from build123d import *

# Parameters (mm, degrees)
SKETCH1_R                 = 2.1
BOSS_EXTRUDE1_DEPTH       = 500
M5X0_8_TAPPED_HOLE1_D     = 4.2
M5X0_8_TAPPED_HOLE1_DEPTH = 13.97
M5X0_8_TAPPED_HOLE1_TIP   = 1.2618073
M5X0_8_TAPPED_HOLE2_D     = 4.2
M5X0_8_TAPPED_HOLE2_DEPTH = 13.97
M5X0_8_TAPPED_HOLE2_TIP   = 1.2618073


with BuildPart() as part:
    # Sketch1 → Boss-Extrude1 (new body)
    with BuildSketch(Plane(origin=(0, 0, 0), x_dir=(-1, 0, 0), z_dir=(0, 0, -1))):
        with BuildLine():
            Line((-3.9, -0.21), (-3.9, -2.839339828))
            Line((-3.9, -2.839339828), (-6.560660172, -5.5))
            Line((-6.560660172, -5.5), (-8.2, -5.5))
            Line((-8.2, -5.5), (-8.2, -3.125))
            Line((-8.2, -3.125), (-8.545, -3.125))
            Line((-8.545, -3.125), (-10, -4.58))
            Line((-10, -4.58), (-10, -9.5))
            ThreePointArc((-10, -9.5), (-9.853553391, -9.853553391), (-9.5, -10))
            Line((-9.5, -10), (-4.58, -10))
            Line((-4.58, -10), (-3.125, -8.545))
            Line((-3.125, -8.545), (-3.125, -8.2))
            Line((-3.125, -8.2), (-5.5, -8.2))
            Line((-5.5, -8.2), (-5.5, -6.560660172))
            Line((-5.5, -6.560660172), (-2.839339828, -3.9))
            Line((-2.839339828, -3.9), (-0.21, -3.9))
            Line((-0.21, -3.9), (0, -3.69))
            Line((0, -3.69), (0.21, -3.9))
            Line((0.21, -3.9), (2.839339828, -3.9))
            Line((2.839339828, -3.9), (5.5, -6.560660172))
            Line((5.5, -6.560660172), (5.5, -8.2))
            Line((5.5, -8.2), (3.125, -8.2))
            Line((3.125, -8.2), (3.125, -8.545))
            Line((3.125, -8.545), (4.58, -10))
            Line((4.58, -10), (9.5, -10))
            ThreePointArc((9.5, -10), (9.853553391, -9.853553391), (10, -9.5))
            Line((10, -9.5), (10, -4.58))
            Line((10, -4.58), (8.545, -3.125))
            Line((8.545, -3.125), (8.2, -3.125))
            Line((8.2, -3.125), (8.2, -5.5))
            Line((8.2, -5.5), (6.560660172, -5.5))
            Line((6.560660172, -5.5), (3.9, -2.839339828))
            Line((3.9, -2.839339828), (3.9, -0.21))
            Line((3.9, -0.21), (3.69, 0))
            Line((3.69, 0), (3.9, 0.21))
            Line((3.9, 0.21), (3.9, 2.839339828))
            Line((3.9, 2.839339828), (6.560660172, 5.5))
            Line((6.560660172, 5.5), (8.2, 5.5))
            Line((8.2, 5.5), (8.2, 3.125))
            Line((8.2, 3.125), (8.545, 3.125))
            Line((8.545, 3.125), (10, 4.58))
            Line((10, 4.58), (10, 9.5))
            ThreePointArc((10, 9.5), (9.853553391, 9.853553391), (9.5, 10))
            Line((9.5, 10), (4.58, 10))
            Line((4.58, 10), (3.125, 8.545))
            Line((3.125, 8.545), (3.125, 8.2))
            Line((3.125, 8.2), (5.5, 8.2))
            Line((5.5, 8.2), (5.5, 6.560660172))
            Line((5.5, 6.560660172), (2.839339828, 3.9))
            Line((2.839339828, 3.9), (0.21, 3.9))
            Line((0.21, 3.9), (0, 3.69))
            Line((0, 3.69), (-0.21, 3.9))
            Line((-0.21, 3.9), (-2.839339828, 3.9))
            Line((-2.839339828, 3.9), (-5.5, 6.560660172))
            Line((-5.5, 6.560660172), (-5.5, 8.2))
            Line((-5.5, 8.2), (-3.125, 8.2))
            Line((-3.125, 8.2), (-3.125, 8.545))
            Line((-3.125, 8.545), (-4.58, 10))
            Line((-4.58, 10), (-9.5, 10))
            ThreePointArc((-9.5, 10), (-9.853553391, 9.853553391), (-10, 9.5))
            Line((-10, 9.5), (-10, 4.58))
            Line((-10, 4.58), (-8.545, 3.125))
            Line((-8.545, 3.125), (-8.2, 3.125))
            Line((-8.2, 3.125), (-8.2, 5.5))
            Line((-8.2, 5.5), (-6.560660172, 5.5))
            Line((-6.560660172, 5.5), (-3.9, 2.839339828))
            Line((-3.9, 2.839339828), (-3.9, 0.21))
            Line((-3.9, 0.21), (-3.69, 0))
            Line((-3.69, 0), (-3.9, -0.21))
        make_face()
        Circle(SKETCH1_R, mode=Mode.SUBTRACT)
    extrude(amount=-BOSS_EXTRUDE1_DEPTH)

    # Split1
    split(bisect_by=Plane.XY.offset(68.2), keep=Keep.TOP)

    # M5x0.8 Tapped Hole1
    with Locations(Plane.XY.offset(500)):
        with Locations((0, 0)):
            Hole(M5X0_8_TAPPED_HOLE1_D / 2, depth=M5X0_8_TAPPED_HOLE1_DEPTH)
            with Locations((0, 0, -(M5X0_8_TAPPED_HOLE1_DEPTH + M5X0_8_TAPPED_HOLE1_TIP / 2))):  # 118° drill point
                Cone(0, M5X0_8_TAPPED_HOLE1_D / 2, M5X0_8_TAPPED_HOLE1_TIP, mode=Mode.SUBTRACT)

    # M5x0.8 Tapped Hole2
    with Locations(Plane(origin=(0, 0, 68.2), x_dir=(-1, 0, 0), z_dir=(0, 0, -1))):
        with Locations((0, 0)):
            Hole(M5X0_8_TAPPED_HOLE2_D / 2, depth=M5X0_8_TAPPED_HOLE2_DEPTH)
            with Locations((0, 0, -(M5X0_8_TAPPED_HOLE2_DEPTH + M5X0_8_TAPPED_HOLE2_TIP / 2))):  # 118° drill point
                Cone(0, M5X0_8_TAPPED_HOLE2_D / 2, M5X0_8_TAPPED_HOLE2_TIP, mode=Mode.SUBTRACT)


solid = part.part
Model file for the job. Use its own axes, mm. Give positions to 0.01 mm unless a question says otherwise; leave off trailing zeros. Write item = value, one per line. Start each with the question number.
1. Two-plate mould, pull along Z, no slides. Class faces 1 (the flat face through (0.1, 2.4, 500)), 2 (the flat face through (-0.1, 2.4, 68.2)): pulls with the +Z half, pulls with the -Z half, needs draft (parallel to the pull), parting line crosses it, or undercut.
2. Drop flat-ended pins along their axis: P1, Ø3, axis at y = -2, z = 374.5, coming from the +X side; P2, Ø1.5, axis at y = 0.5, z = 409, coming from the +X side; P3, Ø0.8, axis at y = 2, z = 222, coming from the -X side; P4, Ø1.9, axis at x = 4.5, z = 373, coming from the -Y side. Give the stop position or say it passes through.
3. Probe line 1 along X through (y, z) = (6.75, 141.5); line 2 along X through (y, z) = (-4.25, 284). List the from-to ranges inside material, lowest first.
Taken from the geometry:
q1.face_1 = pulls with the +Z half
q1.face_2 = pulls with the -Z half
q2.P1 = 8.92
q2.P2 = 3.9
q2.P3 = -3.9
q2.P4 = -10
q3.line_1 = -10 to -5.5, 5.5 to 10
q3.line_2 = -9.67 to -8.2, -5.31 to -3.19, 3.19 to 5.31, 8.2 to 9.67
